Geometry check sheet. Reference: the model listing, model coordinates, mm. A direction names the side the tool comes from. Coordinates: 2 decimals unless noted, no trailing zeros. Write each loop counter-clockwise with the first axis right and the second up, starting at its lowest first coordinate (ties: lowest second). Pieces come first, ordered by that corner, then holes. Notation, with made-up numbers: M -29.5,46.5 L 18.5,46.5 A20 ccw 18.5,63.5 Z; hole C 75,-11.75 d1. An arc over 180 degrees is marked long. Put each result on its own line as item: value. Start each with the question number.
1) Cross-section at A-A on z = 43.5. Record the cut outline in (x, y) (3 decimals).
2) Set-up check for faces 4 (the flat face through (15.9, 11.687, 29.58)), 5 (the flat face through (53, 35, 30)), 6 (the flat face through (11.687, 24.916, 29.58)), 7 (the flat face through (41.313, 24.916, 29.58)): record each of +Z, -Z, +X, -X, +Y, -Y from which the full face is reachable in a straight line by a thin tool's end or side.
3) Scan lines: line 1 along Y through (x, z) = (26.5, 3.5) (3 decimals); line 2 along X through (y, z) = (6, 2); line 3 along Y through (x, z) = (46, 45.5). Record each from-to range of solid material in increasing order.
4) Mould release check, pull along Y, two halves, no side actions. Record for faces 1 (the flat face through (48, 34, 30)), 2 (the flat face through (26, 19, 60)), 3 (the flat face through (26, 0, 30)): released by +Y, released by -Y, zero draft, split by the parting line, or undercut.
5) Gauge pin test, flat ends, axial feed: pin 1 (6 mm diameter, centred on y = 17.5, z = 47, fed in from -X); pin 2 (2 mm diameter, centred on y = 10, z = 20, fed in from -X); pin 3 (5 mm diameter, centred on y = 10.5, z = 45.5, fed in from +X). Record the tip position at first contact, or that the pin passes through.
6) Cross-section at D-D on x = 28.5. Record the cut outline in (y, z).
7) Cross-section at B-B on x = 49. Record the cut outline in (y, z).
8) Cross-section at C-C on y = 13.5. Record the cut outline in (x, z).
Autodesk Inventor part; units mm, degrees
ref_plane "YZ Plane" through (0, 0, 0) normal (1, 0, 0) x (0, 1, 0)
ref_plane "XZ Plane" through (0, 0, 0) normal (0, 1, 0) x (-1, 0, 0)
ref_plane "XY Plane" through (0, 0, 0) normal (0, 0, 1) x (1, 0, 0)
sketch "Sketch1" plane through (0, 0, 0) normal (0, 0, 1) x (1, 0, 0)
  line L0 (0, 0) -> (53, 0)
  line L1 (53, 0) -> (53, 38) construction
  line L2 (53, 38) -> (0, 38)
  line L3 (0, 38) -> (0, 0) construction
  line L4 (5, 35) -> (48, 35)
  line L5 (48, 3) -> (5, 3)
  line L6 (53, 7) -> (0, 7) construction
  line L7 (0, 31) -> (53, 31) construction
  line L8 (5, 38) -> (5, 0) construction
  line L9 (48, 38) -> (48, 0) construction
  line L10 (0, 31) -> (53, 31) construction
  line L11 (0, 31) -> (53, 31) construction
  line L12 (0, 31) -> (54.1143, 31) construction
  line L13 (53, 7) -> (107.1143, 7) construction
  line L14 (0, 31) -> (53.8717, 31) construction
  line L15 (53, 7) -> (106.8717, 7) construction
  line L16 (0, 31) -> (48, 6.0128) construction
  line L17 (0, 31) -> (54.1143, 31) construction
  line L18 (53, 7) -> (5, 31.9872) construction
  line L19 (53, 7) -> (107.1143, 7) construction
  line L20 (53, 38) -> (53, 31)
  line L21 (0, 38) -> (0, 31)
  line L22 (0, 7) -> (0, 0)
  line L23 (53, 7) -> (53, 0)
  line L24 (0, 7) -> (48, 31.9872) construction
  line L25 (0, 7) -> (54.1143, 7) construction
  line L26 (53, 31) -> (5, 6.0128) construction
  line L27 (53, 31) -> (107.1143, 31) construction
  line L28 (5, 35) -> (5, 31.9872)
  line L29 (48, 35) -> (48, 31.9872)
  line L30 (5, 6.0128) -> (5, 3)
  line L31 (48, 6.0128) -> (48, 3)
  line L32 (5, 31.9872) -> (26.5, 20.795)
  line L33 (48, 6.0128) -> (26.5, 17.205)
  line L34 (23.0518, 19) -> (0, 31)
  line L35 (0, 7) -> (23.0518, 19)
  line L36 (26.5, 20.795) -> (48, 31.9872)
  line L37 (26.5, 17.205) -> (5, 6.0128)
  line L38 (29.9482, 19) -> (53, 31)
  line L39 (53, 7) -> (29.9482, 19)
  dimension "d12" = 53
  dimension "d13" = 38
  dimension "d14" = 3
  dimension "d15" = 3
  dimension "d16" = 4
  dimension "d17" = 4
  dimension "d18" = 5
  dimension "d19" = 5
  dimension "d27" = 27.5
  dimension "d28" = 152.5
  dimension "d29" = 27.5
  dimension "d30" = 152.5
extrude "Extrusion1" add sketch "Sketch1" along normal blind 60
sketch "Sketch2" plane through (53, 0, 0) normal (1, 0, 0) x (0, 0, -1)
  circle A0 centre (-55, 5) radius 1.35
  circle A1 centre (-30, 5) radius 1.35
  circle A2 centre (-5, 5) radius 1.35
  circle A3 centre (-36.465, 33) radius 1.35
  circle A4 centre (-11.465, 33) radius 1.35
  point P0 (0, 0)
  dimension "d33" = 2.7
  dimension "d34" = 2.7
  dimension "d35" = 2.7
  dimension "d36" = 2.7
  dimension "d37" = 2.7
properties part number "legspacer_paula_v2"
Answer key:
1. outline: M 0,0 L 53,0 L 53,7 L 29.948,19 L 53,31 L 53,38 L 0,38 L 0,31 L 23.052,19 L 0,7 Z; hole M 5,3 L 48,3 L 48,6.013 L 26.5,17.205 L 5,6.013 Z; hole M 5,31.987 L 26.5,20.795 L 48,31.987 L 48,35 L 5,35 Z
2. face 4: +Z, -Z
2. face 5: +Z, -Z, +X, +Y, -Y
2. face 6: +Z, -Z, -X
2. face 7: +Z, -Z, +X
3. line 1: y = 0 to 3, 17.205 to 20.795, 35 to 38
3. line 2: x = 0 to 5, 48 to 53
3. line 3: y = 0 to 3, 7.05 to 10.64, 27.36 to 30.95, 35 to 38
4. face 1: undercut
4. face 2: zero draft
4. face 3: released by -Y
5. pin 1: stops at x = 14.41
5. pin 2: stops at x = 3.84
5. pin 3: stops at x = 51.08
6. outline: M 0,0 L 3,0 L 3,60 L 0,60 Z; M 16.16,0 L 21.84,0 L 21.84,60 L 16.16,60 Z; M 35,0 L 38,0 L 38,60 L 35,60 Z
7. outline: M 0,0 L 9.08,0 L 9.08,60 L 0,60 Z; M 28.92,0 L 38,0 L 38,60 L 28.92,60 Z
8. outline: M 12.49,0 L 19.38,0 L 19.38,60 L 12.49,60 Z; M 33.62,0 L 40.51,0 L 40.51,60 L 33.62,60 Z
